Here's how the part is built. I have some questions about the finished solid (model axes, mm). A direction names the side the tool comes from. Give positions to 0.01 mm unless a question says otherwise; leave off trailing zeros. Write each loop counter-clockwise with the first axis right and the second up, starting at its lowest first coordinate (ties: lowest second). Pieces come first, ordered by that corner, then holes. Notation, with made-up numbers: (-26, 66) -> (4, 66) arc R17 ccw to (4, 73) -> close; hole circle Ø3 at (8.5, -12). An arc over 180 degrees is marked (long way). Use CSV: the item, a comma, the result in double quotes. Start each with the question number.
(1) Suppose I cut it at B-B on x = 129. List the corners of the cut face in (y, z) for me.
(2) If we mould it in two halves opening along Z, with no side actions, what happens to faces 6 (the flat face through (137, 10, 10)), 7 (the flat face through (152, 10, 18)), 8 (the flat face through (76.077, 54.352, 22.437))? For each: pulls with the +Z half, pulls with the -Z half, needs draft (parallel to the pull), parting line crosses it, or undercut.
(3) Suppose I cut it at A-A on y = 11. List the corners of the cut face in (x, z) for me, plus the area to 3 significant figures.
(4) Suppose I cut it at C-C on z = 5.5. List the corners of the cut face in (x, y) for me.
(5) For pin 1 Ø10.5 at (y, z) = (4.5, 0) entering from +X; pin 2 Ø5 at (y, z) = (9, 20) entering from -X; pin 3 Ø3.5 at (x, y) = (75, 27) entering from +Z, each with a flat end and sliding along its axis, tell me the tip position at first contact or that it passes through.
(6) I need wall thicknesses on L1, parallel to Y at x = 76, z = -9.5; L2, parallel to X at y = 9, z = -8; L3, parallel to Z at x = 26, y = 70. Which ranges of each line are inside material? Lowest first, please. Write a range as [from, to].
(7) Which directions (+Z, -Z, +X, -X, +Y, -Y) give clear straight access to the entire face, cutting with the end or side of a thin tool? Please do faces 1 (the cylindrical face through (-0.636, 40.524, -8.874)), 2 (the flat face through (75, 15, 26)), 3 (the flat face through (70.5, 44, 12)), 4 (the cylindrical face through (120.711, 21.804, -8.874)), 5 (the flat face through (46, 6, 4)).
(8) Suppose I cut it at D-D on x = 63. List the corners of the cut face in (y, z) for me.
Autodesk Inventor part; units mm, degrees
ref_plane "YZ Plane" through (0, 0, 0) normal (1, 0, 0) x (0, 1, 0)
ref_plane "XZ Plane" through (0, 0, 0) normal (0, 1, 0) x (-1, 0, 0)
ref_plane "XY Plane" through (0, 0, 0) normal (0, 0, 1) x (1, 0, 0)
sketch "Sketch1" plane through (0, 0, 0) normal (0, 0, 1) x (1, 0, 0)
  line L0 (0, 0) -> (46, 0)
  line L1 (46, 0) -> (46, 13)
  line L2 (46, 13) -> (106, 13)
  line L3 (106, 13) -> (106, 0)
  line L4 (106, 0) -> (152, 0)
  line L5 (152, 0) -> (152, 20)
  line L6 (152, 20) -> (119, 20)
  line L7 (119, 20) -> (119, 32)
  line L8 (0, 0) -> (0, 20)
  line L9 (0, 20) -> (33, 20)
  line L10 (33, 20) -> (33, 32)
  arc A0 (88.5182, 172.6658) -> (60.9434, 169.5955) centre (76, 159.7315) ccw
  line L11 (88.5182, 172.6658) -> (121.3723, 140.8686)
  arc A1 (-1.0837, 48.545) -> (6.2613, 36.9223) centre (6.0476, 44.9195) ccw
  arc A2 (149, 37.0296) -> (155.0632, 47.9932) centre (147.6772, 44.9195) ccw
  line L12 (60.9434, 169.5955) -> (30.6277, 140.8686)
  line L13 (33, 32) -> (3, 37.5227)
  line L14 (119, 32) -> (149, 37.0296)
  line L15 (155.6101, 45.954) -> (137.729, 112.6291)
  line L16 (-1.9524, 44.9195) -> (14.271, 112.6291)
  arc A3 (137.9006, 111.9892) -> (119.6299, 142.555) centre (76, 95.7315) ccw
  arc A4 (33.3683, 143.4655) -> (13.316, 108.6436) centre (76, 95.7315) ccw
  point P0 (76, 13)
  dimension "d5" = 46
  dimension "d6" = 13
  dimension "d7" = 60
  dimension "d8" = 46
  dimension "d9" = 20
  dimension "d10" = 33
  dimension "d11" = 12
  dimension "d12" = 33
  dimension "d13" = 12
  dimension "d15" = 36
  dimension "d22" = 16
  dimension "d23" = 16
  dimension "d24" = 30
  dimension "d25" = 30
  dimension "d42" = 86
extrude "Extrusion1" add sketch "Sketch1" against normal blind 18 contours L8 L9 L10 L13 A1 L16 A4 L12 A0 L11 A3 L15 A2 L14 L7 L6 L5 L4 L3 L2 L1 L0
sketch "Sketch2" plane through (46, 0, 0) normal (1, 0, 0) x (0, 0, -1)
  point P0 (0, 0)
sketch "Sketch3" plane through (0, 0, 0) normal (0, 0, 1) x (1, 0, 0)
  line L0 (119, 20) -> (152, 20)
  line L1 (0, 20) -> (152, 20)
  line L2 (152, 20) -> (152, 0)
  line L3 (152, 20) -> (152, 0)
  line L4 (152, 0) -> (106, 0)
  line L5 (152, 0) -> (106, 0)
  line L6 (106, 0) -> (106, 13)
  line L7 (106, 0) -> (106, 13)
  line L8 (106, 13) -> (46, 13)
  line L9 (106, 13) -> (46, 13)
  line L10 (46, 13) -> (46, 0)
  line L11 (46, 13) -> (46, 0)
  line L12 (46, 0) -> (0, 0)
  line L13 (46, 0) -> (0, 0)
  line L14 (0, 0) -> (0, 20)
extrude "Extrusion2" add sketch "Sketch3" along normal blind 26
sketch "Sketch4" plane through (33, 20, 0) normal (0, 1, 0) x (1, 0, 0)
  point P0 (-33, 0)
sketch "Sketch5" plane through (152, 0, -18) normal (1, 0, 0) x (0, 0, -1)
  line L0 (0, 0) -> (-44, 0)
  line L1 (-28, 0) -> (-28, 20)
  line L2 (0, 20) -> (-44, 20)
  line L3 (-28, 20) -> (-18, 20)
  line L4 (-18, 20) -> (-18, 0)
  dimension "d32" = 16
  dimension "d33" = 10
extrude "Extrusion3" cut sketch "Sketch5" against normal blind 30
sketch "Sketch6" plane through (0, 0, 0) normal (0, 0, 1) x (1, 0, 0)
  line L0 (119, 20) -> (152, 20)
  point P0 (0, 0)
fillet "Fillet1" radius 4 1 edges at (119, 32, -9)
fillet "Fillet2" radius 6 1 edges at (119, 20, -9)
sketch "Sketch7" plane through (0, 0, -18) normal (-1, 0, 0) x (0, 0, 1)
  line L0 (0, 0) -> (44, 0)
  line L1 (18, 0) -> (18, 20)
  line L2 (18, 20) -> (0, 20)
  line L3 (18, 20) -> (28, 20)
  line L4 (0, 20) -> (44, 20)
  line L5 (28, 20) -> (28, 0)
  dimension "d38" = 18
  dimension "d39" = 10
extrude "Extrusion4" cut sketch "Sketch7" against normal blind 30
sketch "Sketch8" plane through (0, 0, 0) normal (0, 0, 1) x (1, 0, 0)
  point P0 (0, 0)
fillet "Fillet3" radius 8 1 edges at (33, 20, -9)
fillet "Fillet4" radius 2 1 edges at (33, 32, -9)
sketch "Sketch9" plane through (0, 0, 0) normal (0, 0, 1) x (1, 0, 0)
  line L0 (46, 13) -> (106, 13)
  arc A0 (88.5182, 172.6658) -> (60.9434, 169.5955) centre (76, 159.7315) ccw
  line L1 (76, 68) -> (76, 20)
  line L2 (30, 20) -> (122, 20)
  line L3 (76, 20) -> (81.5, 20)
  line L4 (81.5, 20) -> (81.5, 68.6125)
  line L5 (76, 20) -> (70.5, 20)
  line L6 (70.5, 20) -> (70.5, 68.6125)
  line L7 (70.5, 68.6125) -> (81.5, 68.6125)
  point P0 (0, 0)
  point P1 (76, 13)
  point P2 (76, 13)
  point P3 (76, 13)
  point P4 (74.0081, 177.621)
  dimension "d47" = 164.621
  dimension "d49" = 5.5
  dimension "d50" = 5.5
  dimension "d51" = 48
extrude "Extrusion5" add sketch "Sketch9" along normal blind 25
sketch "Sketch10" plane through (0, 0, 0) normal (0, 0, 1) x (1, 0, 0)
  circle A0 centre (76, 169.6287) radius 3.5
  circle A1 centre (145.9486, 44.6297) radius 3.5
  circle A2 centre (8.5813, 44.6297) radius 3.5
  line L0 (81.5, 68.6125) -> (70.5, 68.6125)
  line L1 (122.3386, 32.5597) -> (149, 37.0296)
  line L2 (3, 37.5227) -> (31.3621, 32.3015)
  point P0 (0, 0)
  point P1 (76, 68.6125)
  dimension "d55" = 7
  dimension "d56" = 7
  dimension "d57" = 7
  dimension "d78" = 8
  dimension "d79" = 8
extrude "Extrusion6" cut sketch "Sketch10" against normal blind 25
sketch "Sketch11" plane through (0, 0, 0) normal (0, 0, 1) x (1, 0, 0)
  circle A0 centre (75.9727, 93.6125) radius 25
  line L0 (81.5, 68.6125) -> (70.5, 68.6125)
  point P0 (0, 0)
  point P1 (76, 68.6125)
  dimension "d61" = 50
  dimension "d62" = 25
extrude "Extrusion7" add sketch "Sketch11" along normal blind 40
sketch "Sketch12" plane through (75.9727, 93.6125, 40) normal (0, 0, 1) x (1, 0, 0)
  circle A0 centre (0, 0) radius 17.5
  point P0 (-75.9727, -93.6125)
  dimension "d65" = 35
extrude "Extrusion8" cut sketch "Sketch12" against normal blind 117.25
sketch "Sketch13" plane through (81.5, 20, 0) normal (1, 0, 0) x (0, 0, -1)
  line L0 (0, 48.6125) -> (-40, 48.6125)
  line L1 (-20, 48.6125) -> (-25, 19.3522)
  line L2 (-25, 48.6125) -> (-25, 0)
  line L3 (0, 48.6125) -> (-25, 48.6125)
  line L4 (-20, 48.6125) -> (-25, 48.6125)
  line L5 (-25, 48.6125) -> (-25, 19.3522)
  point P0 (0, -20)
  dimension "d68" = 29.2603
extrude "Extrusion9" cut sketch "Sketch13" against normal blind 15
fillet "Fillet5" radius 4 1 edges at (76, 39.3522, 25)
sketch "Sketch14" plane through (0, 0, 0) normal (0, 0, 1) x (1, 0, 0)
  circle A0 centre (75.9727, 93.6125) radius 25
  arc A1 (70.3554, 69.2518) -> (81.5123, 69.234) centre (75.9727, 93.6125) ccw
  line L0 (70.5, 68.6125) -> (70.3554, 69.2518)
  line L1 (70.4332, 69.234) -> (70.3554, 69.2518)
  line L2 (70.5, 68.6125) -> (75.9727, 68.6125)
  line L3 (70.5, 68.6125) -> (75.9727, 68.6125)
  line L4 (70.5, 68.6125) -> (75.9727, 68.6125)
  point P0 (0, 0)
  point P1 (70.4277, 68.9321)
  dimension "d72" = 25.2956
extrude "Extrusion10" add sketch "Sketch14" along normal blind 20 contours A0 L2 L0
sketch "Sketch15" plane through (0, 0, 0) normal (0, 0, 1) x (1, 0, 0)
  line L0 (81.5, 68.6125) -> (81.5, 39.6866)
  line L1 (81.5, 68.6125) -> (81.5901, 69.2518)
  arc A0 (75.9727, 68.6125) -> (70.3554, 69.2518) centre (75.9727, 93.6125) ccw
  line L2 (75.9727, 68.6125) -> (81.5, 68.6125)
  arc A1 (75.9727, 68.6125) -> (81.5901, 69.2518) centre (75.9727, 93.6125) ccw
  line L3 (81.5, 68.6125) -> (75.9727, 68.6125)
  point P0 (0, 0)
  point P1 (81.545, 68.9321)
  dimension "d75" = 0.3196
extrude "Extrusion11" add sketch "Sketch15" along normal blind 20
properties part number "COMPRESSOR 1" material "Aluminum 6061-AHC"
Geometry says:
1,outline,"(0, -18) -> (20, -18) -> (20, 0) -> (0, 0) -> close; (0, 10) -> (20, 10) -> (20, 26) -> (0, 26) -> close; (33.68, -18) -> (131.61, -18) -> (131.61, 0) -> (33.68, 0) -> close"
2,face 6,"undercut"
2,face 7,"needs draft"
2,face 8,"pulls with the +Z half"
3,outline,"(0, -18) -> (46, -18) -> (46, 26) -> (0, 26) -> (0, 10) -> (30, 10) -> (30, 0) -> (0, 0) -> close; (106, -18) -> (152, -18) -> (152, 0) -> (122, 0) -> (122, 10) -> (152, 10) -> (152, 26) -> (106, 26) -> close"
3,area,"3,450 mm²"
4,outline,"(30, 0) -> (46, 0) -> (46, 13) -> (106, 13) -> (106, 0) -> (122, 0) -> (122, 20) -> (81.5, 20) -> (81.5, 68.61) -> (81.59, 69.25) arc R25 ccw (long way) to (70.36, 69.25) -> (70.5, 68.61) -> (70.5, 20) -> (30, 20) -> close; hole circle Ø35 at (75.97, 93.61)"
5,pin 1,"x = 152"
5,pin 2,"x = 0"
5,pin 3,"z = 25"
6,L1,"[13, 76.11], [111.11, 166.13], [173.13, 177.73]"
6,L2,"[0, 46], [106, 152]"
6,L3,"[-18, 0]"
7,face 1,"+Z, -Z, -X"
7,face 2,"+Z, +X, -X, -Y"
7,face 3,"+Z, -X"
7,face 4,"+Z, -Z, +X"
7,face 5,"+Z, -Z, -Y"
8,outline,"(13, -18) -> (81.87, -18) -> (81.87, 40) -> (72.24, 40) -> (72.24, 0) -> (20, 0) -> (20, 26) -> (13, 26) -> close; (105.36, -18) -> (172.18, -18) -> (172.18, 0) -> (114.98, 0) -> (114.98, 40) -> (105.36, 40) -> close"
